from build123d import *

# Parameters (mm, degrees)
ESTRUSIONE_ESTRUSIONE1_DEPTH = 8
TAGLIO_ESTRUSIONE1_DEPTH     = 1
SCHIZZO4_R                   = 1.75
TAGLIO_ESTRUSIONE2_DEPTH     = 32.448370387
TAGLIO_ESTRUSIONE3_DEPTH     = 1
SCHIZZO6_R                   = 1.75
TAGLIO_ESTRUSIONE4_DEPTH     = 32.448370387
SMUSSO1_SIZE                 = 1.5


with BuildPart() as part:
    # Schizzo1 → Estrusione-Estrusione1 (new body)
    with BuildSketch(Plane.XY):
        Polygon((0, 0), (0, 22), (2, 22), (2, 2), (22, 2), (22, 0), align=None)
    extrude(amount=ESTRUSIONE_ESTRUSIONE1_DEPTH)

    # Schizzo2 → Taglio-Estrusione1 (cut)
    with BuildSketch(Plane(origin=(2, 0, 0), x_dir=(0, 0, -1), z_dir=(1, 0, 0))):
        Polygon((-2.296816706, 15.05), (-0.593633412, 18), (-2.296816706, 20.95), (-5.703183294, 20.95), (-7.406366588, 18), (-5.703183294, 15.05), align=None)
        Polygon((-2.296816706, 6.05), (-0.593633412, 9), (-2.296816706, 11.95), (-5.703183294, 11.95), (-7.406366588, 9), (-5.703183294, 6.05), align=None)
    extrude(amount=-TAGLIO_ESTRUSIONE1_DEPTH, mode=Mode.SUBTRACT)

    # Schizzo4 → Taglio-Estrusione2 (cut, through all)
    with BuildSketch(Plane(origin=(1, 0, 0), x_dir=(0, 0, -1), z_dir=(1, 0, 0))):
        with Locations((-4, 18)):
            Circle(SCHIZZO4_R)
        with Locations((-4, 9)):
            Circle(SCHIZZO4_R)
    extrude(amount=-TAGLIO_ESTRUSIONE2_DEPTH, mode=Mode.SUBTRACT)

    # Schizzo5 → Taglio-Estrusione3 (cut)
    with BuildSketch(Plane(origin=(0, 2, 0), x_dir=(1, 0, 0), z_dir=(0, 1, 0))):
        Polygon((15.05, -5.703183294), (18, -7.406366588), (20.95, -5.703183294), (20.95, -2.296816706), (18, -0.593633412), (15.05, -2.296816706), align=None)
        Polygon((6.05, -5.703183294), (9, -7.406366588), (11.95, -5.703183294), (11.95, -2.296816706), (9, -0.593633412), (6.05, -2.296816706), align=None)
    extrude(amount=-TAGLIO_ESTRUSIONE3_DEPTH, mode=Mode.SUBTRACT)

    # Schizzo6 → Taglio-Estrusione4 (cut, through all)
    with BuildSketch(Plane(origin=(0, 1, 0), x_dir=(1, 0, 0), z_dir=(0, 1, 0))):
        with Locations(Location((18, -4, 0), (0, 0, 270))):
            Circle(SCHIZZO6_R)
        with Locations(Location((9, -4, 0), (0, 0, 270))):
            Circle(SCHIZZO6_R)
    extrude(amount=-TAGLIO_ESTRUSIONE4_DEPTH, mode=Mode.SUBTRACT)

    # Smusso1
    smusso1_edges = [part.edges().sort_by_distance(p)[0] for p in [
        (2, 2, 4),
    ]]
    chamfer(smusso1_edges, length=SMUSSO1_SIZE)


solid = part.part
Input: part model. Units: mm. Frame: model coordinates. A direction names the side the tool comes from. Coordinates: 2 decimals unless noted, no trailing zeros. Loops run counter-clockwise (first coordinate to the right, second up) from the corner with the lowest first, then second, coordinate; pieces in that order, holes last. Notation, with made-up numbers: (12.5, 10.5) -> (37.5, 10.5) arc R21 ccw to (37.5, 26.5) -> close; hole circle Ø11 at (80, -6.75). An arc over 180 degrees is marked (long way). One line per item, written item: value.
(1) Draft query along Z for faces 4 (the face through (0, 11, 4)), 5 (the face through (1.5, 20.95, 4)), 6 (the face through (6, 1, 0)). Return one class per face: pulls with the +Z half, pulls with the -Z half, needs draft (parallel to the pull), parting line crosses it, or undercut.
Answer below:
face 4: needs draft
face 5: undercut
face 6: pulls with the -Z half
(2) Ray query, line 1 along Y through (x, z) = (0.3, 4); line 2 along X through (y, z) = (1.75, 4). Return the intervals inside material, ascending.
Answer below:
line 1: y = 0 to 7.25, 10.75 to 16.25, 19.75 to 22
line 2: x = 0 to 6.05, 11.95 to 15.05, 20.95 to 22
(3) Cut plane D-D (z = 7). Output: boundary loops of the cut face in (x, y), then the cut area to 3 significant figures.
Answer below:
outline: (0, 0) -> (22, 0) -> (22, 2) -> (18.7, 2) -> (18.7, 1) -> (17.3, 1) -> (17.3, 2) -> (9.7, 2) -> (9.7, 1) -> (8.3, 1) -> (8.3, 2) -> (3.5, 2) -> (2, 3.5) -> (2, 8.3) -> (1, 8.3) -> (1, 9.7) -> (2, 9.7) -> (2, 17.3) -> (1, 17.3) -> (1, 18.7) -> (2, 18.7) -> (2, 22) -> (0, 22) -> close
area: 79.5 mm2
(4) Pin query (flat end, axial travel): pin 1 Ø1 at (y, z) = (16, 1.5) entering from +X; pin 2 Ø1.5 at (y, z) = (3, 4.5) entering from +X; pin 3 Ø4.5 at (x, z) = (17.5, 5.5) entering from +Y. Return the tip coordinate at first contact, or that it passes through.
Answer below:
pin 1: stops at x = 2
pin 2: stops at x = 3.25
pin 3: stops at y = 2
(5) Set-up query: faces 1 (the face through (1.5, 11.95, 4)), 2 (the face through (2, 13, 4)), 3 (the face through (7.55, 1.51, 1.43)). Return all of +Z, -Z, +X, -X, +Y, -Y with unobstructed straight access to the full face (end or side cutting, diameter ignored); none if empty.
Answer below:
face 1: +X
face 2: +Z, -Z, +X, +Y
face 3: +Y
(6) Cut plane C-C (z = 4). Give the number of separate pieces and of enclosed holes in the cut face, then the cut area to 3 significant figures.
Answer below:
separate pieces: 5
enclosed holes: 0
area: 47.5 mm2
(7) Cut plane A-A (y = 17). Output: boundary loops of the cut face in (x, z).
Answer below:
outline: (0, 0) -> (2, 0) -> (2, 1.17) -> (1, 1.17) -> (1, 2.56) -> (0, 2.56) -> close; (0, 5.44) -> (1, 5.44) -> (1, 6.83) -> (2, 6.83) -> (2, 8) -> (0, 8) -> close
